```python
from build123d import *

# Parameters (mm, degrees)
SKETCH1_R           = 3
BOSS_EXTRUDE1_DEPTH = 3
CHAMFER1_SIZE       = 0.3
CUT_EXTRUDE1_DEPTH  = 2.5
CHAMFER2_SIZE       = 0.3
SKETCH3_R           = 1.5
BOSS_EXTRUDE2_DEPTH = 6
CHAMFER3_SIZE       = 0.2


with BuildPart() as part:
    # Sketch1 → Boss-Extrude1 (new body)
    with BuildSketch(Plane(origin=(0, 0, 0), x_dir=(1, 0, 0), z_dir=(0, 1, 0))):
        with Locations(Location((0, 0, 0), (0, 0, 270))):  # turned: the seam where the file's is
            Circle(SKETCH1_R)
    extrude(amount=BOSS_EXTRUDE1_DEPTH)

    # Chamfer1
    chamfer1_edges = [part.edges().sort_by_distance(p)[0] for p in [
        (0, 3, -3),
    ]]
    chamfer(chamfer1_edges, length=CHAMFER1_SIZE)

    # Sketch2 → Cut-Extrude1 (cut)
    with BuildSketch(Plane(origin=(0, 3, 0), x_dir=(1, 0, 0), z_dir=(0, 1, 0))):
        Polygon((1.732050808, 0), (0.866025404, 1.5), (-0.866025404, 1.5), (-1.732050808, 0), (-0.866025404, -1.5), (0.866025404, -1.5), align=None)
    extrude(amount=-CUT_EXTRUDE1_DEPTH, mode=Mode.SUBTRACT)

    # Chamfer2
    chamfer2_edges = [part.edges().sort_by_distance(p)[0] for p in [
        (1.299038106, 3, 0.75),
        (1.299038106, 3, -0.75),
        (0, 3, -1.5),
        (-1.299038106, 3, -0.75),
        (-1.299038106, 3, 0.75),
        (0, 3, 1.5),
    ]]
    chamfer(chamfer2_edges, length=CHAMFER2_SIZE)

    # Sketch3 → Boss-Extrude2 (add)
    with BuildSketch(Plane.XZ):
        with Locations(Location((0, 0, 0), (0, 0, 90))):  # turned: the seam where the file's is
            Circle(SKETCH3_R)
    extrude(amount=BOSS_EXTRUDE2_DEPTH)

    # Chamfer3
    chamfer3_edges = [part.edges().sort_by_distance(p)[0] for p in [
        (0, -6, -1.5),
    ]]
    chamfer(chamfer3_edges, length=CHAMFER3_SIZE)


solid = part.part
```
The listing builds one solid part. Answer for the finished solid, in the listing's coordinates (mm). A direction names the side the tool comes from. Coordinates: 2 decimals unless noted, no trailing zeros. Loops run counter-clockwise (first coordinate to the right, second up) from the corner with the lowest first, then second, coordinate; pieces in that order, holes last. Notation, with made-up numbers: (-7.5, 81.25) - (31.5, 81.25) arc R22 cw to (31.5, 98.25) - close; hole circle Ø10 at (6, 63.5). An arc over 180 degrees is marked (long way). Write item = value, one per line.
1) This flat-tipped pin is pushed along its axis until it touches: P1, Ø3, axis at y = -3, z = 0, coming from the -X side. Where does it stop, or does it pass through?
Responses:
P1 = -1.5
2) Section A-A (y = 1) is taken. Determine the outline of the cut face in (x, z).
Responses:
outline = circle Ø6 at (0, 0); hole (-1.73, 0) - (-0.87, -1.5) - (0.87, -1.5) - (1.73, 0) - (0.87, 1.5) - (-0.87, 1.5) - close
3) Section C-C (y = -1) is taken. Determine the outline of the cut face in (x, z).
Responses:
outline = circle Ø3 at (0, 0)
4) Determine the mould class of faces 4 (the face through (0, -6, 0)), 5 (the face through (-0.45, -2.86, 1.43)), 6 (the face through (-1.434, 2.848, 0.811)) for opening direction Z: pulls with the +Z half, pulls with the -Z half, needs draft (parallel to the pull), parting line crosses it, or undercut.
Responses:
face_4 = needs draft
face_5 = parting line crosses it
face_6 = undercut
5) Section B-B (x = 0) is taken. Determine the outline of the cut face in (y, z), plus the area to 3 significant figures.
Responses:
outline = (-6, -1.3) - (-5.8, -1.5) - (0, -1.5) - (0, -3) - (2.7, -3) - (3, -2.7) - (3, -1.8) - (2.7, -1.5) - (0.5, -1.5) - (0.5, 1.5) - (2.7, 1.5) - (3, 1.8) - (3, 2.7) - (2.7, 3) - (0, 3) - (0, 1.5) - (-5.8, 1.5) - (-6, 1.3) - close
area = 28.3 mm^2
6) Find the intervals of material crossed by line 1 along Z through (x, y) = (-0.05, -2.5); line 2 along Z through (x, y) = (2.4, 1.75); line 3 along Y through (x, z) = (-1.2, 1.7), in increasing order.
Responses:
line_1 = -1.5 to 1.5
line_2 = -1.8 to 1.8
line_3 = 0 to 3
7) Which of the six approach directions +Z, -Z, +X, -X, +Y, -Y give full straight-line access (tool end or side, diameter ignored) to faces 1 (the face through (1.42, 2.85, 0.84)), 2 (the face through (-1.3, 0, 1.3)), 3 (the face through (-2, 3, -1))?
Responses:
face_1 = +Y
face_2 = -Y
face_3 = +Z, -Z, +X, -X, +Y
